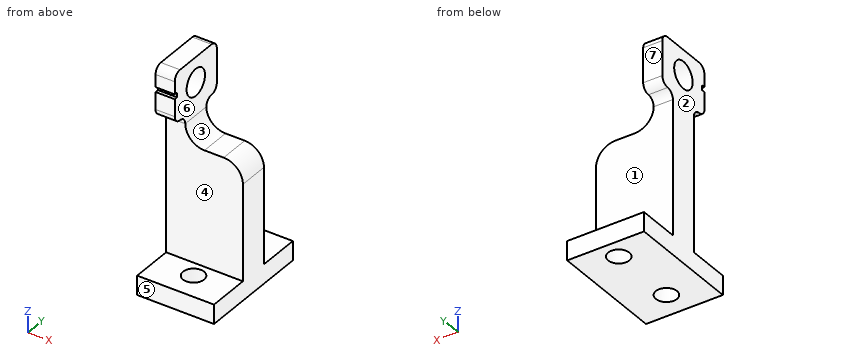
```python
from build123d import *

# Parameters (mm, degrees)
SKETCH1_R               = 2.75
BOSS_EXTRUDE1_DEPTH     = 5
SKETCH2_W               = 20
SKETCH2_H               = 4
BOSS_EXTRUDE2_DEPTH     = 50
CUT_EXTRUDE1_DEPTH      = 73.479956342
CUT_EXTRUDE1_DEPTH_BACK = 73.479956342
SKETCH5_W               = 15
SKETCH5_H               = 8
CUT_EXTRUDE2_DEPTH      = 15
SKETCH6_W               = 15
SKETCH6_H               = 8
CUT_EXTRUDE3_DEPTH      = 5
FILLET1_R               = 5
SKETCH7_W               = 13
SKETCH7_H               = 4
BOSS_EXTRUDE3_DEPTH     = 5
SKETCH8_R               = 3.5
CUT_EXTRUDE5_DEPTH      = 73.479956342
SKETCH9_W               = 1.25
SKETCH9_H               = 0.9
SKETCH9_H_2             = 0.5
CUT_EXTRUDE6_DEPTH      = 5
FILLET2_R               = 2


with BuildPart() as part:
    # Sketch1 → Boss-Extrude1 (new body)
    with BuildSketch(Plane.XY):
        Polygon((15, -12.759140208), (25, -12.759140208), (25, -42.759140208), (5, -42.759140208), (5, -12.759140208), align=None)
        with Locations((15, -35.919713403)):
            Circle(SKETCH1_R, mode=Mode.SUBTRACT)
        with Locations((15, -17.759140208)):
            Circle(SKETCH1_R, mode=Mode.SUBTRACT)
    extrude(amount=BOSS_EXTRUDE1_DEPTH)

    # Sketch2 → Boss-Extrude2 (add)
    with BuildSketch(Plane.XY.offset(5)):
        with Locations((15, -25.759140208)):
            Rectangle(SKETCH2_W, SKETCH2_H)
        with Locations((15, -29.759140208)):
            Rectangle(SKETCH2_W, SKETCH2_H)
    extrude(amount=BOSS_EXTRUDE2_DEPTH)

    # Sketch3 → Cut-Extrude1 (cut, two sides: drawn at the far end of the back side and taken through both)
    with BuildSketch(Plane(origin=(25, 0, 0), x_dir=(0, 0, -1), z_dir=(1, 0, 0)).offset(-CUT_EXTRUDE1_DEPTH_BACK)):
        with BuildLine():
            Line((-46.695516884, -26.87718455), (-48.490552878, -27.759140208))
            Line((-48.490552878, -27.759140208), (-46.490552878, -27.759140208))
            ThreePointArc((-46.490552878, -27.759140208), (-46.542467666, -27.306410701), (-46.695516884, -26.87718455))
        make_face()
        with BuildLine():
            Line((-50.490552878, -27.759140208), (-48.490552878, -27.759140208))
            Line((-48.490552878, -27.759140208), (-46.695516884, -26.87718455))
            ThreePointArc((-46.695516884, -26.87718455), (-48.943282385, -25.811054996), (-50.490552878, -27.759140208))
        make_face()
        with BuildLine():
            Line((-46.490552878, -27.759140208), (-48.490552878, -27.759140208))
            Line((-48.490552878, -27.759140208), (-50.490552878, -27.759140208))
            ThreePointArc((-50.490552878, -27.759140208), (-48.490552878, -29.759140208), (-46.490552878, -27.759140208))
        make_face()
    extrude(amount=CUT_EXTRUDE1_DEPTH + CUT_EXTRUDE1_DEPTH_BACK, mode=Mode.SUBTRACT)

    # Sketch5 → Cut-Extrude2 (cut)
    with BuildSketch(Plane.XY.offset(55)):
        with Locations((17.5, -27.759140208)):
            Rectangle(SKETCH5_W, SKETCH5_H)
    extrude(amount=-CUT_EXTRUDE2_DEPTH, mode=Mode.SUBTRACT)

    # Sketch6 → Cut-Extrude3 (cut)
    with BuildSketch(Plane.XY.offset(40)):
        with Locations((17.5, -27.759140208)):
            Rectangle(SKETCH6_W, SKETCH6_H)
    extrude(amount=-CUT_EXTRUDE3_DEPTH, mode=Mode.SUBTRACT)

    # Fillet1
    fillet1_edges = [part.edges().sort_by_distance(p)[0] for p in [
        (10, -27.759140208, 35),
        (25, -27.759140208, 35),
    ]]
    fillet(fillet1_edges, radius=FILLET1_R)

    # Sketch7 → Boss-Extrude3 (add)
    with BuildSketch(Plane.ZY.offset(-5)):
        with Locations((48.5, -33.759140208)):
            Rectangle(SKETCH7_W, SKETCH7_H)
        with Locations((48.5, -21.759140208)):
            Rectangle(SKETCH7_W, SKETCH7_H)
    extrude(amount=-BOSS_EXTRUDE3_DEPTH)

    # Sketch8 → Cut-Extrude5 (cut, through all)
    with BuildSketch(Plane.ZY.offset(-5)):
        with Locations(Location((48.490552878, -27.759140208, 0), (0, 0, 270))):
            Circle(SKETCH8_R)
    extrude(amount=-CUT_EXTRUDE5_DEPTH, mode=Mode.SUBTRACT)

    # Sketch9 → Cut-Extrude6 (cut)
    with BuildSketch(Plane.ZY.offset(-5)):
        with Locations((49.115552878, -35.309140208)):
            Rectangle(SKETCH9_W, SKETCH9_H)
        with Locations((47.865552878, -36.009140208)):
            Rectangle(SKETCH9_W, SKETCH9_H_2)
        with Locations((49.115552878, -36.009140208)):
            Rectangle(SKETCH9_W, SKETCH9_H_2)
    extrude(amount=-CUT_EXTRUDE6_DEPTH, mode=Mode.SUBTRACT)

    # Fillet2
    fillet2_edges = [part.edges().sort_by_distance(p)[0] for p in [
        (7.5, -23.759140208, 42),
        (7.5, -31.759140208, 42),
        (7.5, -35.759140208, 42),
        (7.5, -19.759140208, 42),
        (7.5, -19.759140208, 55),
        (7.5, -35.759140208, 55),
    ]]
    fillet(fillet2_edges, radius=FILLET2_R - 0.0001)  # a hair under: the kernel refuses the full size


solid = part.part
```
Verification items for the finished model (mm, model axes). Face numbers are marked on the shaded views. A direction names the side the tool comes from. Give positions to 0.01 mm unless a question says otherwise; leave off trailing zeros. Order: outer loops, then holes, each group sorted by start corner. A loop starts at its lowest first (then second) coordinate and runs counter-clockwise, first axis right, second up. Notation, with made-up numbers: M 15,-26.5 L 38,-26.5 A7 cw 38,-18.5 Z; hole C 30.25,-5.75 d6. An arc over 180 degrees is marked long. Answer in a Markdown table with one row per item. Add a question column.
Item 1: Scan lines: probe 1 along Y at (x, z) = (15, 3.2); probe 2 along Z at (x, y) = (18.5, -35.5); probe 3 along Z at (x, y) = (20.25, -28.5). Record each from-to range of solid material in increasing order. Write a range as from..to.
Item 2: Tool access check on the marked faces 5, 6 and 7. Record the directions out of +Z, -Z, +X, -X, +Y, -Y that give a thin tool (end or side, any length) a straight path to the whole face; none if there is none.
Item 3: Section check B-B, the plane x = 18.5. Enter the section's corners in (y, z), and give its area (3 significant figures).
Item 4: Gauge pin test, flat ends, axial feed: pin 1 (0.6 mm diameter, centred on x = 7.5, z = 49.5, fed in from -Y); pin 2 (5 mm diameter, centred on x = 9.5, z = 14.5, fed in from -Y); pin 3 (2 mm diameter, centred on x = 17, y = -31, fed in from +Z). Record the tip position at first contact, or that the pin passes through.
Item 5: Section check D-D, the plane x = 15.75. Enter the section's corners in (y, z).
Item 6: Section check A-A, the plane y = -28.75. Enter the section's corners in (x, z), and give its area (3 significant figures).
Item 7: Section check C-C, the plane z = 10. Enter the section's corners in (x, y).
Item 8: Mould release check, pull along Z, two halves, no side actions. Record for the marked faces 1, 2, 3 and 4: released by +Z, released by -Z, zero draft, split by the parting line, or undercut.
Filled sheet:
| question | item | result |
|---|---|---|
| 1 | probe 1 | y = -42.76..-38.67, -33.17..-20.51, -15.01..-12.76 |
| 1 | probe 2 | z = 0..5 |
| 1 | probe 3 | z = 0..34.99 |
| 2 | face 5 | +Z, -Z, +X, -X, -Y |
| 2 | face 6 | +Z, +X, +Y, -Y |
| 2 | face 7 | +Z, +X, -X, +Y |
| 3 | outline | M -42.76,0 L -12.76,0 L -12.76,5 L -23.76,5 L -23.76,35 L -31.76,35 L -31.76,5 L -42.76,5 Z |
| 3 | area | 390 mm^2 |
| 4 | pin 1 | stops at y = -35.76 |
| 4 | pin 2 | stops at y = -31.76 |
| 4 | pin 3 | stops at z = 35 |
| 5 | outline | M -42.76,0 L -38.57,0 L -38.57,5 L -42.76,5 Z; M -33.27,0 L -20.4,0 L -20.4,5 L -23.76,5 L -23.76,35 L -31.76,35 L -31.76,5 L -33.27,5 Z; M -15.11,0 L -12.76,0 L -12.76,5 L -15.11,5 Z |
| 6 | outline | M 5,0 L 25,0 L 25,30 A5 ccw 20,35 L 15,35 A5 cw 10,40 L 10,45.13 L 5,45.13 Z; M 5,51.85 L 10,51.85 L 10,55 L 5,55 Z |
| 6 | area | 766 mm^2 |
| 7 | outline | M 5,-31.76 L 25,-31.76 L 25,-23.76 L 5,-23.76 Z |
| 8 | face 1 | undercut |
| 8 | face 2 | zero draft |
| 8 | face 3 | released by +Z |
| 8 | face 4 | undercut |
